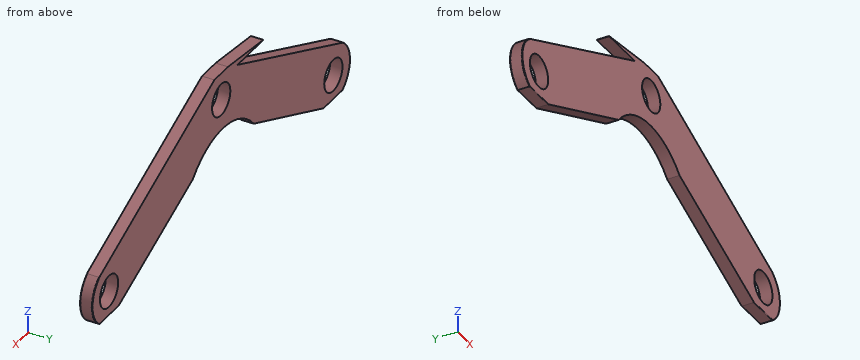
from build123d import *

# Parameters (mm, degrees)
F0_R     = 6.5
F1_DEPTH = 5
F3_R     = 0.2


# Not quite as in the source:
# - a feature of the source that left no trace in its solid (it failed there, or was rolled back) is left out


with BuildPart() as f1:
    # F0 (on Front) → F1 (new body)
    with BuildSketch(Plane.XZ):
        with BuildLine():
            Line((-11.6401047196, 31.2017867216), (-86.9632974703, -2.0251641974))
            ThreePointArc((-86.9632974703, -2.0251641974), (-91.998328651, -11.9984870467), (-86.6332495807, -21.7982132784))
            Line((-86.6332495807, -21.7982132784), (-73.3667504193, -21.7982132784))
            Line((-73.3667504193, -21.7982132784), (-23.2548427581, 0))
            ThreePointArc((-23.2548427581, 0), (-1.8189642808, 10.5340546664), (20.2171359245, 1.3213741908))
            Line((20.2171359245, 1.3213741908), (73.3667504193, -21.7982132784))
            Line((73.3667504193, -21.7982132784), (86.6332495807, -21.7982132784))
            ThreePointArc((86.6332495807, -21.7982132784), (91.998328651, -11.9984870467), (86.9632974703, -2.0251641974))
            Line((86.9632974703, -2.0251641974), (4.8428413091, 34.2017867216))
            Line((4.8428413091, 34.2017867216), (-4.8393128322, 34.2017867216))
            Line((-4.8393128322, 34.2017867216), (-30, 31.3017867216))
            Line((-30, 31.3017867216), (-30, 31.2017867216))
            Line((-30, 31.2017867216), (-11.6401047196, 31.2017867216))
        make_face()
        with Locations((-80, -11.7982132784)):
            Circle(F0_R, mode=Mode.SUBTRACT)
        with Locations((80, -11.7982132784)):
            Circle(F0_R, mode=Mode.SUBTRACT)
        with Locations((0, 23.2017867216)):
            Circle(F0_R, mode=Mode.SUBTRACT)
    extrude(amount=F1_DEPTH)

    # F3
    f3_edges = [f1.edges().sort_by_distance(p)[0] for p in [
        (80, -5, -21.798213),
        (80, 0, -21.798213),
        (-80, -5, -21.798213),
        (-80, 0, -21.798213),
        (-86.63325, -2.5, -21.798213),
        (-91.998329, 0, -11.998487),
        (-91.998329, -5, -11.998487),
        (86.63325, -2.5, -21.798213),
        (91.998329, 0, -11.998487),
        (91.998329, -5, -11.998487),
    ]]
    fillet(f3_edges, radius=F3_R)


solid = f1.part
Could you check a few things on this model? Use its own coordinates, in mm. Round coordinates to 2 decimals unless told otherwise and drop trailing zeros. Write each loop counter-clockwise with the first axis right and the second up, starting at its lowest first coordinate (ties: lowest second). Pieces come first, ordered by that corner, then holes. Notation, with made-up numbers: (-38, 56) - (-14, 56) arc R18 ccw to (-14, 77) - close; hole circle Ø5 at (9.25, 70). An arc over 180 degrees is marked (long way). Put each result on its own line as item: value. Start each with the question number.
(1) I want a section at B-B, the plane y = -2. Please give me the cut outline in (x, z), plus the area to 3 significant figures.
(2) Will these pins go through, and if not, where does the flat tip stop? pin 1 (1.5 mm diameter, centred on x = -55.5, y = -2.5, fed in from -Z); pin 2 (11.5 mm diameter, centred on x = 0, z = 23.2, fed in from +Y); pin 3 (1.5 mm diameter, centred on x = -20, y = -3, fed in from -Z); pin 4 (2 mm diameter, centred on x = 44, y = -4, fed in from +Z).
(3) I want a section at C-C, the plane z = 8. Please give me the cut outline in (x, y), plus the area to 3 significant figures.
(4) I need wall thicknesses on probe 1 along Z at (x, y) = (0, -0.95); probe 2 along X at (y, z) = (-2.5, -14.5); probe 3 along Z at (x, y) = (80, -3.65). Which ranges of each line are inside material? Lowest first, please.
(5) I want a section at A-A, the plane x = -25. Please give me the cut outline in (y, z), plus the area to 3 significant figures.
(6) I want a section at D-D, the plane x = -77. Please give me the cut outline in (y, z), plus the area to 3 significant figures.
Here are the results:
1. outline: (-86.96, -2.03) arc R12 ccw to (-86.68, -21.76) arc R0.2 ccw to (-86.57, -21.8) - (-73.37, -21.8) - (-23.25, 0) arc R28.88 cw to (20.22, 1.32) - (73.37, -21.8) - (86.57, -21.8) arc R0.2 ccw to (86.68, -21.76) arc R12 ccw to (86.96, -2.03) - (4.84, 34.2) - (-4.84, 34.2) - (-30, 31.3) - (-30, 31.2) - (-11.64, 31.2) - close; hole circle Ø13 at (-80, -11.8); hole circle Ø13 at (0, 23.2); hole circle Ø13 at (80, -11.8)
1. area: 4,100 mm^2
2. pin 1: stops at z = -14.35
2. pin 2: passes through
2. pin 3: stops at z = 2.68
2. pin 4: stops at z = 17.37
3. outline: (-64.24, -5) - (-12.8, -5) - (-12.8, 0) - (-64.24, 0) - close; (10.92, -5) - (64.24, -5) - (64.24, 0) - (10.92, 0) - close
3. area: 524 mm^2
4. probe 1: z = 10.53 to 16.7, 29.7 to 34.2
4. probe 2: x = -91.69 to -85.91, -74.09 to -56.59, 56.59 to 74.09, 85.91 to 91.69
4. probe 3: z = -21.8 to -18.3, -5.3 to 1.05
5. outline: (-5, -0.76) - (0, -0.76) - (0, 25.31) - (-5, 25.31) - close; (-5, 31.2) - (0, 31.2) - (0, 31.88) - (-5, 31.88) - close
5. area: 134 mm^2
6. outline: (-5, -21.6) arc R0.2 ccw to (-4.8, -21.8) - (-0.2, -21.8) arc R0.2 ccw to (0, -21.6) - (0, -17.56) - (-5, -17.56) - close; (-5, -6.03) - (0, -6.03) - (0, 2.37) - (-5, 2.37) - close
6. area: 63.2 mm^2
